Build history of the part. All positions in model axes, mm. Face numbers are marked on the shaded views. A direction names the side the tool comes from. Give positions to 0.01 mm unless a question says otherwise; leave off trailing zeros. Order: outer loops, then holes, each group sorted by start corner. A loop starts at its lowest first (then second) coordinate and runs counter-clockwise, first axis right, second up. Notation, with made-up numbers: (27, 48.25) - (54, 48.25) arc R8 cw to (54, 63.25) - close; hole circle Ø10 at (18, -4.5). An arc over 180 degrees is marked (long way). Answer in a Markdown table with one row per item.
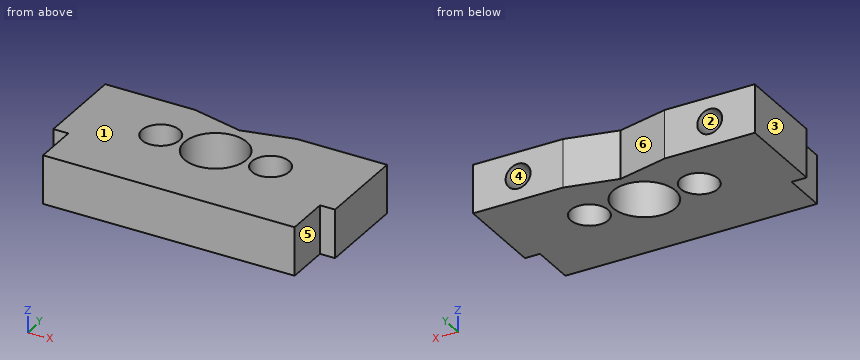
Autodesk Inventor part; units mm, degrees
ref_plane "YZ Plane" through (0, 0, 0) normal (1, 0, 0) x (0, 1, 0)
ref_plane "XZ Plane" through (0, 0, 0) normal (0, 1, 0) x (-1, 0, 0)
ref_plane "XY Plane" through (0, 0, 0) normal (0, 0, 1) x (1, 0, 0)
sketch "Sketch1" plane through (0, 0, 0) normal (0, 0, 1) x (1, 0, 0)
  point P0 (0, 0)
sketch "Sketch2" plane through (0, 0, 0) normal (0, 0, 1) x (1, 0, 0)
  line L0 (-22.9271, 6.1236) -> (-22.9271, -16.8764)
  line L1 (-22.9271, -16.8764) -> (48.9029, -16.8764)
  line L2 (48.9029, -16.8764) -> (48.9029, 6.1236)
  line L3 (48.9029, 6.1236) -> (-22.9271, 6.1236)
  point P0 (0, 0)
  dimension "d0" = 23
  dimension "d1" = 71.83
extrude "Extrusion1" add sketch "Sketch2" against normal blind 12.36
sketch "Sketch3" plane through (0, 0, 0) normal (0, 0, 1) x (1, 0, 0)
  point P0 (0, 0)
sketch "Sketch4" plane through (0, 0, 0) normal (0, 0, 1) x (1, 0, 0)
  line L0 (0.0479, 6.1236) -> (25.9279, 6.1236)
  line L1 (25.9279, 6.1236) -> (12.9879, 3.1378)
  line L2 (12.9879, 3.1378) -> (0.0479, 6.1236)
  line L3 (48.9029, 6.1236) -> (-22.9271, 6.1236)
  line L4 (48.9029, -16.8764) -> (48.9029, 6.1236)
  circle A0 centre (12.9879, -7.3764) radius 7.9375
  circle A1 centre (-1.0121, -7.3764) radius 4.7625
  circle A2 centre (26.9879, -7.3764) radius 4.7625
  line L5 (-22.9271, -16.8764) -> (48.9029, -16.8764)
  line L6 (-19.0821, -16.8764) -> (45.0579, -16.8764)
  line L7 (45.0579, -16.8764) -> (45.0579, -28.1264)
  line L8 (45.0579, -28.1264) -> (-19.0821, -28.1264)
  line L9 (-19.0821, -28.1264) -> (-19.0821, -16.8764)
  line L10 (-22.9271, 6.1236) -> (-22.9271, -16.8764)
  point P0 (0, 0)
  dimension "d4" = 25.88
  dimension "d7" = 13.28
  dimension "d8" = 0
  dimension "d10" = 2.9858
  dimension "d11" = 35.915
  dimension "d12" = 15.875
  dimension "d13" = 9.5
  dimension "d14" = 14
  dimension "d15" = 9.5
  dimension "d16" = 9.5
  dimension "d17" = 14
  dimension "d18" = 9.525
  dimension "d19" = 9.525
  dimension "d20" = 64.14
  dimension "d21" = 11.25
  dimension "d22" = 3.845
  dimension "d23" = 0
extrude "Extrusion2" cut sketch "Sketch4" against normal blind 12.36 contours L0 L1 L2 | A0 | A1 | A2
extrude "Extrusion3" add sketch "Sketch4" against normal blind 12.36 contours L5 L7 L8 L9
sketch "Sketch5" plane through (-22.9271, 6.1236, 0) normal (0, 1, 0) x (1, 0, 0)
  circle A0 centre (11.4875, 6.18) radius 3.175
  line L0 (0, 12.36) -> (22.975, 12.36)
  line L1 (0, 0) -> (0, 12.36)
  circle A1 centre (60.342, 6.18) radius 3.175
  line L2 (71.83, 0) -> (71.83, 12.36)
  point P0 (22.9271, 0)
  dimension "d28" = 6.18
  dimension "d29" = 6.35
  dimension "d30" = 11.4875
  dimension "d31" = 6.35
  dimension "d32" = 11.488
extrude "Extrusion4" cut sketch "Sketch5" against normal blind 13
thread "Thread1"
properties part number "rod holder on"
1. Cut at A-A on x = 29. Write the cut outline in (y, z).
Check result:
| item | result |
|---|---|
| outline | (-28.13, -12.36) - (-11.69, -12.36) - (-11.69, 0) - (-28.13, 0) - close; (-3.06, -12.36) - (6.12, -12.36) - (6.12, 0) - (-3.06, 0) - close |
2. Cut at C-C on z = -11. Write the cut outline in (x, y) (1 decimal), and give its area (3 significant figures).
Check result:
| item | result |
|---|---|
| outline | (-22.9, -16.9) - (-19.1, -16.9) - (-19.1, -28.1) - (45.1, -28.1) - (45.1, -16.9) - (48.9, -16.9) - (48.9, 6.1) - (25.9, 6.1) - (13, 3.1) - (0, 6.1) - (-22.9, 6.1) - close; hole circle Ø9.5 at (-1, -7.4); hole circle Ø15.9 at (13, -7.4); hole circle Ø9.5 at (27, -7.4) |
| area | 1,990 mm² |
3. Probe line 1 (X direction, y = 1, z = -3.5); line 2 (X direction, y = -4, z = -12); line 3 (X direction, y = -2.5, z = -7). List the from-to ranges inside material, lowest first.
Check result:
| item | result |
|---|---|
| line 1 | x = -22.93 to -13.14, -9.74 to 35.71, 39.12 to 48.9 |
| line 2 | x = -22.93 to -4.37, 2.35 to 5.8, 20.17 to 23.63, 30.35 to 48.9 |
| line 3 | x = -22.93 to -14.51, -8.37 to 6.72, 19.25 to 34.35, 40.48 to 48.9 |
4. Two-plate mould, pull along X, no slides. Class the marked faces 1, 2 and 3: +X half, -X half, draft (parallel to the pull), parting line (faces both ways), or undercut.
Check result:
| item | result |
|---|---|
| face 1 | draft |
| face 2 | undercut |
| face 3 | -X half |
5. Cut at B-B on y = -4. Write the cut outline in (x, z) (3 decimals).
Check result:
| item | result |
|---|---|
| outline | (-22.927, -12.36) - (-4.371, -12.36) - (-4.371, 0) - (-22.927, 0) - close; (2.347, -12.36) - (5.804, -12.36) - (5.804, 0) - (2.347, 0) - close; (20.171, -12.36) - (23.629, -12.36) - (23.629, 0) - (20.171, 0) - close; (30.347, -12.36) - (48.903, -12.36) - (48.903, 0) - (30.347, 0) - close; hole circle Ø6.35 at (-11.44, -6.18); hole circle Ø6.35 at (37.415, -6.18) |
6. Cut at D-D on x = 11.5. Write the cut outline in (y, z).
Check result:
| item | result |
|---|---|
| outline | (-28.13, -12.36) - (-15.17, -12.36) - (-15.17, 0) - (-28.13, 0) - close; (0.42, -12.36) - (3.48, -12.36) - (3.48, 0) - (0.42, 0) - close |
7. Which spindle directions (+Z, -Z, +X, -X, +Y, -Y) get a long thin tool onto all of the face, cutting with end or side? Do the marked faces 4, 5 and 6. Say none if no direction does.
Check result:
| item | result |
|---|---|
| face 4 | +Y |
| face 5 | +Z, -Z, +X, -Y |
| face 6 | +Z, -Z, +Y |
